Verification items for this drawing (mm, ordinates from the low corner). Give positions to 0.01 mm unless a question says otherwise; leave off trailing zeros. Order: outer loops, then holes, each group sorted by start corner. A loop starts at its lowest first (then second) coordinate and runs counter-clockwise, first axis right, second up.
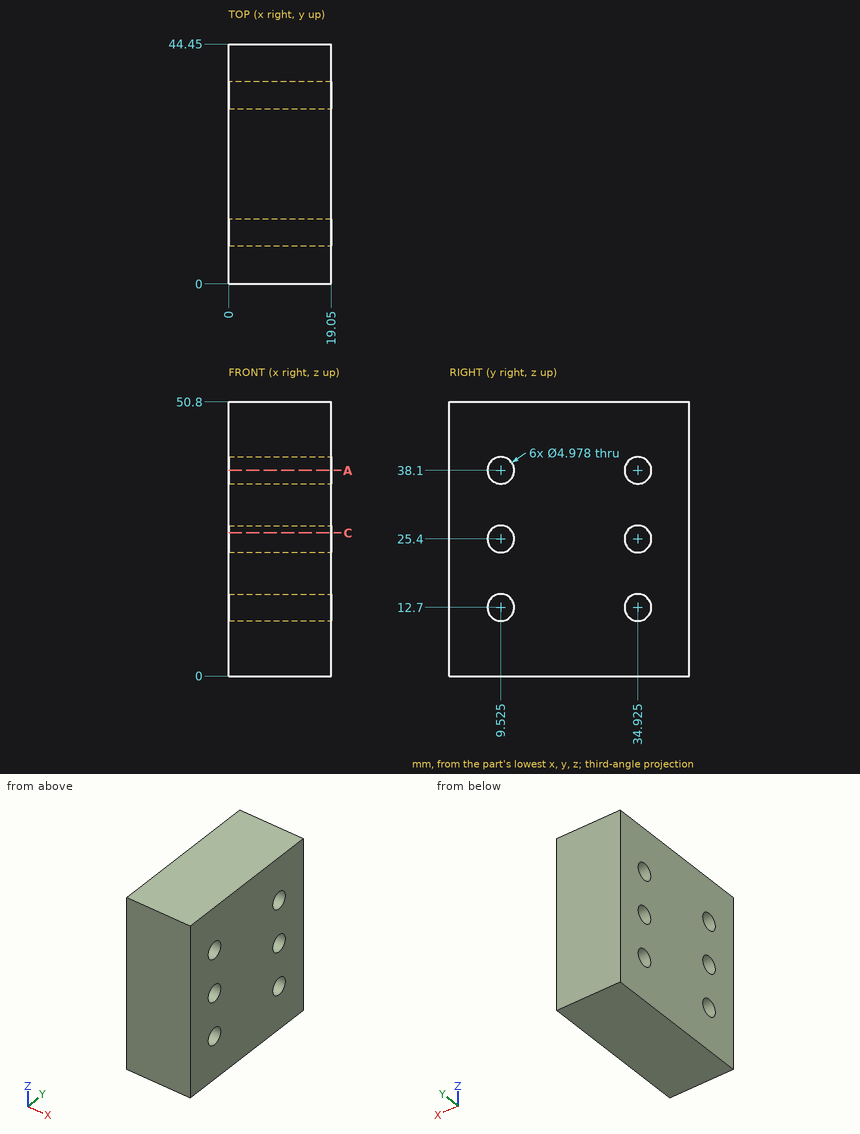
Q1. Cross-section at A-A, the plane z = 38.1. Give the number of separate pieces and of enclosed holes in the cut face, and give its area (3 significant figures).
Q2. Cross-section at C-C, the plane z = 26.5. Record the boundary of the cut face in (x, y).
Q3. Thickness scan on L1, parallel to Z at x = 7.75, y = 35; L2, parallel to Z at x = 5.75, y = 8; L3, parallel to Y at x = 17.75, z = 25. Record the ranges inside material, lowest first.
Answers follow:
1. separate pieces: 3
1. enclosed holes: 0
1. area: 657 mm2
2. outline: (0, 0) - (19.05, 0) - (19.05, 7.29) - (0, 7.29) - close; (0, 11.76) - (19.05, 11.76) - (19.05, 32.69) - (0, 32.69) - close; (0, 37.16) - (19.05, 37.16) - (19.05, 44.45) - (0, 44.45) - close
3. L1: z = 0 to 10.21, 15.19 to 22.91, 27.89 to 35.61, 40.59 to 50.8
3. L2: z = 0 to 10.73, 14.67 to 23.43, 27.37 to 36.13, 40.07 to 50.8
3. L3: y = 0 to 7.07, 11.98 to 32.47, 37.38 to 44.45
